Build history of the part. All positions in model axes, mm. Give positions to 0.01 mm unless a question says otherwise; leave off trailing zeros. Order: outer loops, then holes, each group sorted by start corner. A loop starts at its lowest first (then second) coordinate and runs counter-clockwise, first axis right, second up. Notation, with made-up numbers: (-13.5, 55.5) - (8.5, 55.5) arc R30 ccw to (8.5, 94.5) - close; hole circle Ø8 at (23, 1). An arc over 180 degrees is marked (long way). Write each question's results on one line, items separated by ' | '. Start each with the question number.
1) Drill centre lines: line 1 along Y through (x, z) = (-8.5, 1.5); line 2 along Y through (x, z) = (-6.5, 2.7); line 3 along Y through (x, z) = (-114, 0.95). Where is each one in solid material? Low to high. Write a range as from..to.
2) Drop flat-ended pins along their axis: pin 1 Ø1 at (x, z) = (92, 2) entering from +Y; pin 2 Ø1.5 at (y, z) = (55, 0.5) entering from -X. Give the stop position or say it passes through.
3) Cut at D-D on y = -41. List the corners of the cut face in (x, z).
4) Cut at A-A on y = 39. List the corners of the cut face in (x, z).
5) Cut at B-B on y = -118. List the corners of the cut face in (x, z).
6) Cut at C-C on z = 1.6. State how many separate pieces and enclosed holes the cut face has, plus the area to 3 significant figures.
7) Two-plate mould, pull along X, no slides. Class faces 1 (the face through (-35.769, -161.076, 1.479)), 2 (the face through (-2, -34, 3)), 3 (the face through (57.8, 56.65, 1.48)): +X half, -X half, draft (parallel to the pull), parting line (faces both ways), or undercut.
from build123d import *

# Parameters (mm, degrees)
SKETCH11_R          = 165
SKETCH11_R_2        = 1.6
SKETCH11_R_3        = 37.5
SKETCH11_R_4        = 20
BOSS_EXTRUDE4_DEPTH = 3


with BuildPart() as part:
    # Sketch11 → Boss-Extrude4 (new body)
    with BuildSketch(Plane.XY):
        Circle(SKETCH11_R)
        with Locations((-48, 110)):
            Circle(SKETCH11_R_2, mode=Mode.SUBTRACT)
        with Locations((0, 158)):
            Circle(SKETCH11_R_2, mode=Mode.SUBTRACT)
        with Locations((48, 110)):
            Circle(SKETCH11_R_2, mode=Mode.SUBTRACT)
        with Locations((0, 62)):
            Circle(SKETCH11_R_2, mode=Mode.SUBTRACT)
        with Locations((71.262794416, 96.569219382)):
            Circle(SKETCH11_R_2, mode=Mode.SUBTRACT)
        with Locations((136.832013798, 79)):
            Circle(SKETCH11_R_2, mode=Mode.SUBTRACT)
        with Locations((119.262794416, 13.430780618)):
            Circle(SKETCH11_R_2, mode=Mode.SUBTRACT)
        with Locations((53.693575035, 31)):
            Circle(SKETCH11_R_2, mode=Mode.SUBTRACT)
        with Locations((119.262794416, -13.430780618)):
            Circle(SKETCH11_R_2, mode=Mode.SUBTRACT)
        with Locations((136.832013798, -79)):
            Circle(SKETCH11_R_2, mode=Mode.SUBTRACT)
        with Locations((71.262794416, -96.569219382)):
            Circle(SKETCH11_R_2, mode=Mode.SUBTRACT)
        with Locations((53.693575035, -31)):
            Circle(SKETCH11_R_2, mode=Mode.SUBTRACT)
        with Locations((48, -110)):
            Circle(SKETCH11_R_2, mode=Mode.SUBTRACT)
        with Locations((0, -158)):
            Circle(SKETCH11_R_2, mode=Mode.SUBTRACT)
        with Locations((-48, -110)):
            Circle(SKETCH11_R_2, mode=Mode.SUBTRACT)
        with Locations((0, -62)):
            Circle(SKETCH11_R_2, mode=Mode.SUBTRACT)
        with Locations((-71.262794416, -96.569219382)):
            Circle(SKETCH11_R_2, mode=Mode.SUBTRACT)
        with Locations((-136.832013798, -79)):
            Circle(SKETCH11_R_2, mode=Mode.SUBTRACT)
        with Locations((-119.262794416, -13.430780618)):
            Circle(SKETCH11_R_2, mode=Mode.SUBTRACT)
        with Locations((-53.693575035, -31)):
            Circle(SKETCH11_R_2, mode=Mode.SUBTRACT)
        with Locations((-119.262794416, 13.430780618)):
            Circle(SKETCH11_R_2, mode=Mode.SUBTRACT)
        with Locations((-136.832013798, 79)):
            Circle(SKETCH11_R_2, mode=Mode.SUBTRACT)
        with Locations((-71.262794416, 96.569219382)):
            Circle(SKETCH11_R_2, mode=Mode.SUBTRACT)
        with Locations((-53.693575035, 31)):
            Circle(SKETCH11_R_2, mode=Mode.SUBTRACT)
        with Locations((0, 110)):
            Circle(SKETCH11_R_3, mode=Mode.SUBTRACT)
        with Locations((95.262794416, 55)):
            Circle(SKETCH11_R_3, mode=Mode.SUBTRACT)
        with Locations((95.262794416, -55)):
            Circle(SKETCH11_R_3, mode=Mode.SUBTRACT)
        with Locations((0, -110)):
            Circle(SKETCH11_R_3, mode=Mode.SUBTRACT)
        with Locations((-95.262794416, -55)):
            Circle(SKETCH11_R_3, mode=Mode.SUBTRACT)
        with Locations((-95.262794416, 55)):
            Circle(SKETCH11_R_3, mode=Mode.SUBTRACT)
        Circle(SKETCH11_R_4, mode=Mode.SUBTRACT)
    extrude(amount=BOSS_EXTRUDE4_DEPTH)


solid = part.part
Results:
1) line 1: -164.78..-146.52, -73.48..-18.1, 18.1..73.48, 146.52..164.78 | line 2: -164.87..-146.93, -73.07..-18.91, 18.91..73.07, 146.93..164.87 | line 3: -119.29..-87.48, -22.52..22.52, 87.48..119.29
2) pin 1: y = 137.31 | pin 2: x = -155.83
3) outline: (-159.82, 0) - (-130.05, 0) - (-130.05, 3) - (-159.82, 3) - close; (-60.47, 0) - (60.47, 0) - (60.47, 3) - (-60.47, 3) - close; (130.05, 0) - (159.82, 0) - (159.82, 3) - (130.05, 3) - close
4) outline: (-160.32, 0) - (-129.18, 0) - (-129.18, 3) - (-160.32, 3) - close; (-61.35, 0) - (61.35, 0) - (61.35, 3) - (-61.35, 3) - close; (129.18, 0) - (160.32, 0) - (160.32, 3) - (129.18, 3) - close
5) outline: (-115.33, 0) - (-36.64, 0) - (-36.64, 3) - (-115.33, 3) - close; (36.64, 0) - (115.33, 0) - (115.33, 3) - (36.64, 3) - close
6) separate pieces: 1 | enclosed holes: 31 | area: 57,600 mm^2
7) face 1: parting line | face 2: draft | face 3: undercut
